```python
from build123d import *

# Parameters (mm, degrees)
F1_DEPTH = 1
F3_DEPTH = 55
F5_DEPTH = 10


with BuildPart() as f1:
    # F0 (on Top) → F1 (new body)
    with BuildSketch(Plane.XY):
        with BuildLine():
            Line((-72, -40), (72, -40))
            ThreePointArc((72, -40), (84.727922, -34.727922), (90, -22))
            Line((90, -22), (90, 22))
            ThreePointArc((90, 22), (84.727922, 34.727922), (72, 40))
            Line((72, 40), (-72, 40))
            ThreePointArc((-72, 40), (-84.727922, 34.727922), (-90, 22))
            Line((-90, 22), (-90, -22))
            ThreePointArc((-90, -22), (-84.727922, -34.727922), (-72, -40))
        make_face()
        with BuildLine():
            Line((-72, 30), (72, 30))
            ThreePointArc((72, 30), (77.656854, 27.656854), (80, 22))
            Line((80, 22), (80, -22))
            ThreePointArc((80, -22), (77.656854, -27.656854), (72, -30))
            Line((72, -30), (-72, -30))
            ThreePointArc((-72, -30), (-77.656854, -27.656854), (-80, -22))
            Line((-80, -22), (-80, 22))
            ThreePointArc((-80, 22), (-77.656854, 27.656854), (-72, 30))
        make_face(mode=Mode.SUBTRACT)
    extrude(amount=F1_DEPTH)

    # F2 (on face) → F3 (join)
    with BuildSketch(Plane.XY.offset(1)):
        with BuildLine():
            Line((81.6, -22), (81.6, 22))
            ThreePointArc((81.6, 22), (78.788225, 28.788225), (72, 31.6))
            Line((72, 31.6), (-72, 31.6))
            ThreePointArc((-72, 31.6), (-78.788225, 28.788225), (-81.6, 22))
            Line((-81.6, 22), (-81.6, -22))
            ThreePointArc((-81.6, -22), (-78.788225, -28.788225), (-72, -31.6))
            Line((-72, -31.6), (72, -31.6))
            ThreePointArc((72, -31.6), (78.788225, -28.788225), (81.6, -22))
        make_face()
        with BuildLine():
            Line((-72, 30), (72, 30))
            ThreePointArc((72, 30), (77.656854, 27.656854), (80, 22))
            Line((80, 22), (80, -22))
            ThreePointArc((80, -22), (77.656854, -27.656854), (72, -30))
            Line((72, -30), (-72, -30))
            ThreePointArc((-72, -30), (-77.656854, -27.656854), (-80, -22))
            Line((-80, -22), (-80, 22))
            ThreePointArc((-80, 22), (-77.656854, 27.656854), (-72, 30))
        make_face(mode=Mode.SUBTRACT)
    extrude(amount=F3_DEPTH)

    # F4 (on face) → F5 (join)
    with BuildSketch(Plane(origin=(0, 0, 0), x_dir=(1, 0, 0), z_dir=(0, 0, -1))):
        with BuildLine():
            ThreePointArc((-78.692388, -31.192388), (-78.882689, -30.23568), (-79.424621, -29.424621))
            Line((-79.424621, -29.424621), (-82.960155, -32.960155))
            ThreePointArc((-82.960155, -32.960155), (-80.23568, -33.502087), (-78.692388, -31.192388))
        make_face()
        with BuildLine():
            Line((-82.960155, -32.960155), (-79.424621, -29.424621))
            ThreePointArc((-79.424621, -29.424621), (-82.960155, -29.424621), (-82.960155, -32.960155))
        make_face()
        with BuildLine():
            ThreePointArc((83.692388, -31.192388), (82.149097, -28.882689), (79.424621, -29.424621))
            Line((79.424621, -29.424621), (82.960155, -32.960155))
            ThreePointArc((82.960155, -32.960155), (83.502087, -32.149097), (83.692388, -31.192388))
        make_face()
        with BuildLine():
            Line((82.960155, -32.960155), (79.424621, -29.424621))
            ThreePointArc((79.424621, -29.424621), (79.424621, -32.960155), (82.960155, -32.960155))
        make_face()
        with BuildLine():
            ThreePointArc((82.960155, 32.960155), (79.424621, 32.960155), (79.424621, 29.424621))
            Line((79.424621, 29.424621), (82.960155, 32.960155))
        make_face()
        with BuildLine():
            Line((82.960155, 32.960155), (79.424621, 29.424621))
            ThreePointArc((79.424621, 29.424621), (82.149097, 28.882689), (83.692388, 31.192388))
            ThreePointArc((83.692388, 31.192388), (83.502087, 32.149097), (82.960155, 32.960155))
        make_face()
        with BuildLine():
            ThreePointArc((-82.960155, 32.960155), (-82.960155, 29.424621), (-79.424621, 29.424621))
            Line((-79.424621, 29.424621), (-82.960155, 32.960155))
        make_face()
        with BuildLine():
            Line((-82.960155, 32.960155), (-79.424621, 29.424621))
            ThreePointArc((-79.424621, 29.424621), (-78.882689, 30.23568), (-78.692388, 31.192388))
            ThreePointArc((-78.692388, 31.192388), (-80.23568, 33.502087), (-82.960155, 32.960155))
        make_face()
    extrude(amount=-F5_DEPTH)


solid = f1.part
```
The model under review builds one solid part; all positions refer to its coordinate system, in mm. A direction names the side the tool comes from. Coordinates: 2 decimals unless noted, no trailing zeros. Loops run counter-clockwise (first coordinate to the right, second up) from the corner with the lowest first, then second, coordinate; pieces in that order, holes last. Notation, with made-up numbers: (74, 39) -> (109, 39) arc R10 cw to (109, 58) -> close; hole circle Ø4 at (51.25, 3). An arc over 180 degrees is marked (long way). Answer as CSV lines item,"result".
Item 1: Take a section at A-A, the plane y = -10.5. State the section outline as (x, z) points.
Results below:
outline,"(-90, 0) -> (-80, 0) -> (-80, 56) -> (-81.6, 56) -> (-81.6, 1) -> (-90, 1) -> close; (80, 0) -> (90, 0) -> (90, 1) -> (81.6, 1) -> (81.6, 56) -> (80, 56) -> close"
Item 2: Take a section at C-C, the plane z = 45.5. State the section outline as (x, y) points, and give its area (3 significant figures).
Results below:
outline,"(-81.6, -22) arc R9.6 ccw to (-72, -31.6) -> (72, -31.6) arc R9.6 ccw to (81.6, -22) -> (81.6, 22) arc R9.6 ccw to (72, 31.6) -> (-72, 31.6) arc R9.6 ccw to (-81.6, 22) -> close; hole (-80, -22) arc R8 ccw to (-72, -30) -> (72, -30) arc R8 ccw to (80, -22) -> (80, 22) arc R8 ccw to (72, 30) -> (-72, 30) arc R8 ccw to (-80, 22) -> close"
area,"690 mm2"
Item 3: Machinability: for faces 4 (the flat face through (-1, -31.6, 28)), 5 (the cylindrical face through (77.719, -27.594, 27.608)), 6 (the flat face through (-81.6, 0, 28)), which of the approach directions +Z, -Z, +X, -X, +Y, -Y give a long, thin tool a straight path to every point of the face, cutting with its end or side? Answer none if there is none.
Results below:
face 4,"+Z, -Y"
face 5,"+Z, -Z"
face 6,"+Z, -X"
Item 4: For L1, parallel to Y at x = -41.5, z = 43.5; L2, parallel to X at y = -21, z = 26.5; L3, parallel to X at y = -26, z = 24, list the stretches that pass through material, from the lowest coordinate up.
Results below:
L1,"y = -31.6 to -30, 30 to 31.6"
L2,"x = -81.6 to -80, 80 to 81.6"
L3,"x = -80.73 to -78.93, 78.93 to 80.73"
Item 5: Draft analysis for pull direction X (two halves, no side actions). For faces 1 (the flat face through (-7, 33, 1)), 2 (the flat face through (81.6, 0, 28)), 3 (the flat face through (81, 31, 10)), state which applies: +X half, -X half, draft (parallel to the pull), parting line (faces both ways), or undercut.
Results below:
face 1,"undercut"
face 2,"+X half"
face 3,"draft"
Item 6: Insertion check: pin 1 (5.5 mm diameter, centred on x = -80.5, y = -32, fed in from +Z); pin 2 (1 mm diameter, centred on y = -3.5, z = 47, fed in from +X); pin 3 (17 mm diameter, centred on x = 18, z = 25, fed in from +Y). Each pin has a flat end and moves straight along its axis. Give the tip position at first contact, or say it passes through.
Results below:
pin 1,"stops at z = 10"
pin 2,"stops at x = 81.6"
pin 3,"stops at y = 31.6"
Item 7: Take a section at B-B, the plane x = 25. State the section outline as (y, z) points.
Results below:
outline,"(-40, 0) -> (-30, 0) -> (-30, 56) -> (-31.6, 56) -> (-31.6, 1) -> (-40, 1) -> close; (30, 0) -> (40, 0) -> (40, 1) -> (31.6, 1) -> (31.6, 56) -> (30, 56) -> close"
